Check sheet for the drawn part. Datum: minimum x, y, z corner. Units: mm. Coordinates: 2 decimals unless noted, no trailing zeros. Loops run counter-clockwise (first coordinate to the right, second up) from the corner with the lowest first, then second, coordinate; pieces in that order, holes last.
Q1. Go/stop test with flat-tipped pins: P1, Ø3, axis at x = 84.85, z = 20, coming from the +Y side; P2, Ø0.5, axis at x = 34.5, y = 0.5, coming from the +Z side; P3, Ø6, axis at x = 14.5, z = 34, coming from the +Y side; P4, Ø5.5, axis at x = 4.58, z = 85.09, coming from the -Y side. Record where each tip stops, or that it passes through.
Q2. Material ranges on probe 1 along Z at (x, y) = (90.31, 1.05); probe 2 along X at (y, z) = (0.55, 9.58); probe 3 along X at (y, z) = (0.4, 7.62), recorded low to high.
Q3. Sectioned sample at A-A (x = 53). Enter the section's corners in (y, z).
Q4. Sectioned sample at B-B (z = 20). Enter the section's corners in (x, y).
Q5. Sectioned sample at C-C (z = 85.09). Enter the section's corners in (x, y).
Q6. Sectioned sample at D-D (y = 3.25). Enter the section's corners in (x, z).
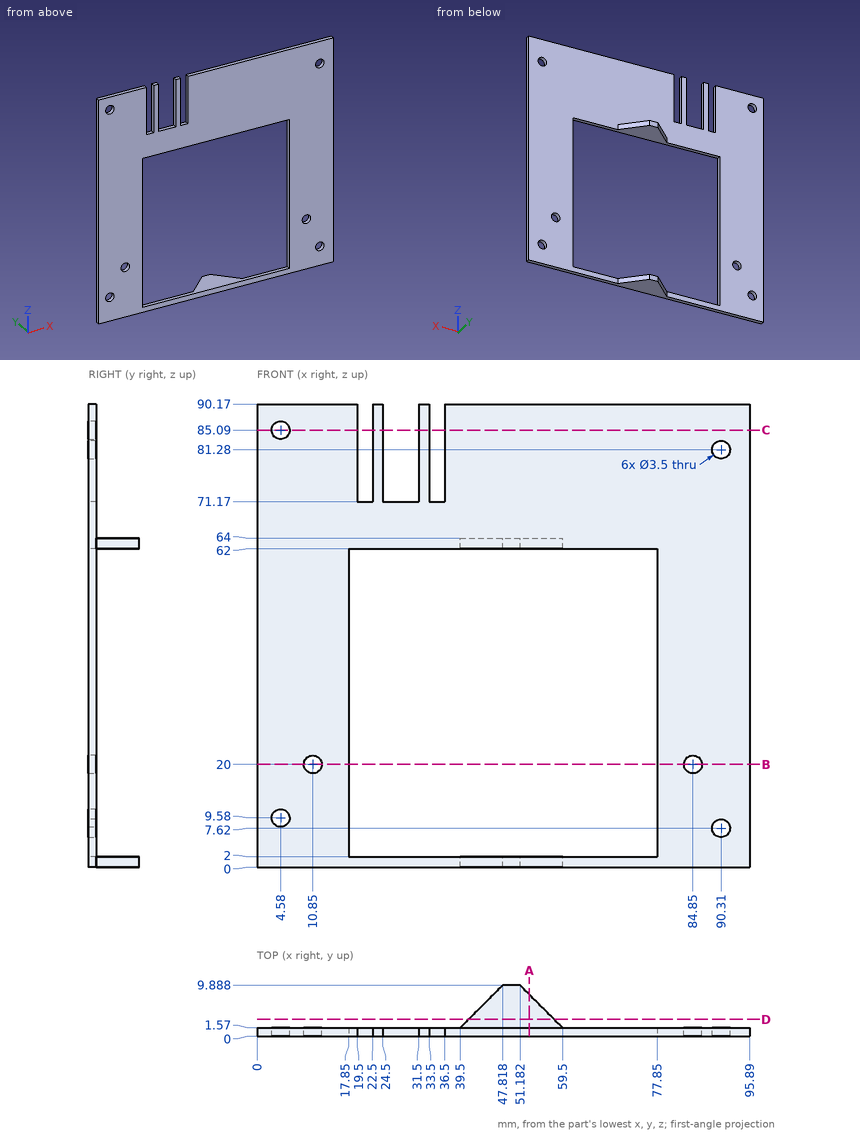
Geometry check:
1. P1: passes through
1. P2: stops at z = 71.17
1. P3: stops at y = 1.57
1. P4: stops at y = 0
2. probe 1: z = 0 to 5.87, 9.37 to 79.53, 83.03 to 90.17
2. probe 2: x = 0 to 2.83, 6.33 to 17.85, 77.85 to 95.89
2. probe 3: x = 0 to 17.85, 77.85 to 88.56, 92.06 to 95.89
3. outline: (0, 0) - (8.07, 0) - (8.07, 2) - (0, 2) - close; (0, 62) - (8.07, 62) - (8.07, 64) - (1.57, 64) - (1.57, 90.17) - (0, 90.17) - close
4. outline: (0, 0) - (9.1, 0) - (9.1, 1.57) - (0, 1.57) - close; (12.6, 0) - (17.85, 0) - (17.85, 1.57) - (12.6, 1.57) - close; (77.85, 0) - (83.1, 0) - (83.1, 1.57) - (77.85, 1.57) - close; (86.6, 0) - (95.89, 0) - (95.89, 1.57) - (86.6, 1.57) - close
5. outline: (0, 0) - (2.83, 0) - (2.83, 1.57) - (0, 1.57) - close; (6.33, 0) - (19.5, 0) - (19.5, 1.57) - (6.33, 1.57) - close; (22.5, 0) - (24.5, 0) - (24.5, 1.57) - (22.5, 1.57) - close; (31.5, 0) - (33.5, 0) - (33.5, 1.57) - (31.5, 1.57) - close; (36.5, 0) - (95.89, 0) - (95.89, 1.57) - (36.5, 1.57) - close
6. outline: (41.18, 0) - (57.82, 0) - (57.82, 2) - (41.18, 2) - close; (41.18, 62) - (57.82, 62) - (57.82, 64) - (41.18, 64) - close
